CAD build for the part. Positions are in the model's coordinates, mm. Round coordinates to 2 decimals unless told otherwise and drop trailing zeros. Order: outer loops, then holes, each group sorted by start corner. A loop starts at its lowest first (then second) coordinate and runs counter-clockwise, first axis right, second up.
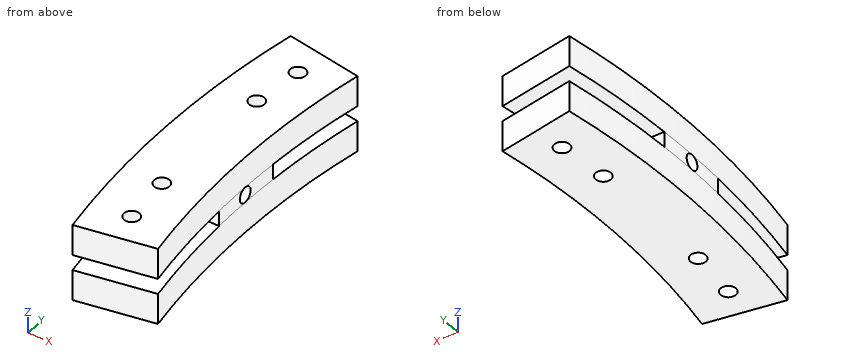
```python
from build123d import *

# Parameters (mm, degrees)
BOSS_EXTRUDE3_DEPTH   = 7.5
CUT_EXTRUDE4_DEPTH    = 1.5
BOSS_EXTRUDE5_DEPTH   = 1.5
SKETCH4_R             = 3
BEARING_HOLE_DEPTH    = 1.25
SHAFT_HOLE_DEPTH      = 33.837885572
SHAFT_HOLE_DEPTH_BACK = 33.837885572
SKETCH7_R             = 1.5
SKETCH3_R             = 1.5
MOUNT_HOLE_DEPTH      = 178.777126728


with BuildPart() as part:
    # Sketch1 → Boss-Extrude3 (new, symmetric)
    with BuildSketch(Plane.XY):
        with BuildLine():
            Line((-157.569240482, 27.783708427), (-172.341356777, 30.388431092))
            ThreePointArc((-172.341356777, 30.388431092), (-175, 0), (-172.341356777, -30.388431092))
            Line((-172.341356777, -30.388431092), (-157.569240482, -27.783708427))
            ThreePointArc((-157.569240482, -27.783708427), (-160, 0), (-157.569240482, 27.783708427))
        make_face()
    extrude(amount=BOSS_EXTRUDE3_DEPTH, both=True)

    # Sketch1_6 → Cut-Extrude4 (cut, symmetric)
    with BuildSketch(Plane.XY):
        with BuildLine():
            Line((-157.569240482, 27.783708427), (-172.341356777, 30.388431092))
            ThreePointArc((-172.341356777, 30.388431092), (-175, 0), (-172.341356777, -30.388431092))
            Line((-172.341356777, -30.388431092), (-157.569240482, -27.783708427))
            ThreePointArc((-157.569240482, -27.783708427), (-160, 0), (-157.569240482, 27.783708427))
        make_face()
    extrude(amount=CUT_EXTRUDE4_DEPTH, both=True, mode=Mode.SUBTRACT)


with BuildPart() as cut_extrude4_piece_1:
    # of the separate pieces the step leaves, piece 1, a body of its own (cut_extrude4_pieces)
    add(part.part.solids().sort_by_distance((-172.341356777, 30.388431092, -1.5))[0])



with BuildPart() as cut_extrude4_piece_2:
    # of the separate pieces the step leaves, piece 2, a body of its own (cut_extrude4_pieces)
    add(part.part.solids().sort_by_distance((-172.341356777, 30.388431092, 7.5))[0])


with BuildPart() as cut_extrude4_piece_1_1:
    add(cut_extrude4_piece_1.part)

    add(cut_extrude4_piece_2.part)  # Boss-Extrude5 merges Cut-Extrude4 piece 2
    # Sketch6 → Boss-Extrude5 (add, symmetric)
    with BuildSketch(Plane.XY):
        with BuildLine():
            Line((-159.824122084, 7.5), (-174.839211849, 7.5))
            ThreePointArc((-174.839211849, 7.5), (-175, 0), (-174.839211849, -7.5))
            Line((-174.839211849, -7.5), (-159.824122084, -7.5))
            ThreePointArc((-159.824122084, -7.5), (-160, 0), (-159.824122084, 7.5))
        make_face()
    extrude(amount=BOSS_EXTRUDE5_DEPTH, both=True)

    # Sketch4 → bearing hole (cut, symmetric)
    with BuildSketch(Plane(origin=(-167.5, 0, 0), x_dir=(0, 0, -1), z_dir=(1, 0, 0))):
        Circle(SKETCH4_R)
    extrude(amount=BEARING_HOLE_DEPTH, both=True, mode=Mode.SUBTRACT)

    # Sketch7 → shaft hole (cut, two sides: drawn at the far end of the back side and taken through both)
    with BuildSketch(Plane(origin=(-167.5, 0, 0), x_dir=(0, 0, -1), z_dir=(1, 0, 0)).offset(-SHAFT_HOLE_DEPTH_BACK)):
        Circle(SKETCH7_R)
    extrude(amount=SHAFT_HOLE_DEPTH + SHAFT_HOLE_DEPTH_BACK, mode=Mode.SUBTRACT)

    # Sketch3 → mount hole (cut, symmetric)
    with BuildSketch(Plane(origin=(0, 0, 0), x_dir=(-1, 0, 0), z_dir=(0, 0, -1))):
        with Locations((165.891323638, 23.158556552)):
            Circle(SKETCH3_R)
        with Locations((166.977667312, 13.217738807)):
            Circle(SKETCH3_R)
    mount_hole = extrude(amount=MOUNT_HOLE_DEPTH, both=True, mode=Mode.SUBTRACT)

    # Mirror1: mount hole across plane
    add(mount_hole.mirror(Plane.ZX), mode=Mode.SUBTRACT)


solid = cut_extrude4_piece_1_1.part
```
1. Pin check, flat tips, straight feed: P1, Ø5, axis at y = 9, z = -5.5, coming from the -X side; P2, Ø4, axis at y = 13.5, z = -3, coming from the -X side; P3, Ø3.5, axis at x = -167, z = 0.5, coming from the +Y side. Stop position of each tip, or through.
2. Cut at D-D, the plane z = 4. Write the cut outline in (x, y), and give its area (3 significant figures).
3. Cut at A-A, the plane y = -9.5. Write the cut outline in (x, z).
4. Drill centre lines: line 1 (Y direction, x = -165.75, z = 3.5); line 2 (Y direction, x = -167, z = 6); line 3 (Z direction, x = -168.25, y = -9). Where is each one in solid material? Low to high.
5. Cut at C-C, the plane y = 9. Write the cut outline in (x, z), and give its area (3 significant figures).
6. Cut at B-B, the plane z = 0. Write the cut outline in (x, y).
Outcome:
1. P1: stops at x = -174.88
1. P2: stops at x = -174.62
1. P3: stops at y = 29.7
2. outline: (-172.34, -30.39) - (-157.57, -27.78) arc R160 cw to (-157.57, 27.78) - (-172.34, 30.39) arc R175 ccw to start; hole circle Ø3 at (-166.98, -13.22); hole circle Ø3 at (-166.98, 13.22); hole circle Ø3 at (-165.89, -23.16); hole circle Ø3 at (-165.89, 23.16)
2. area: 849 mm2
3. outline: (-174.74, -7.5) - (-159.72, -7.5) - (-159.72, -1.5) - (-174.74, -1.5) - close; (-174.74, 1.5) - (-159.72, 1.5) - (-159.72, 7.5) - (-174.74, 7.5) - close
4. line 1: y = -29.23 to -24.65, -21.67 to -14.08, -12.36 to 12.36, 14.08 to 21.67, 24.65 to 29.23
4. line 2: y = -29.45 to -24.17, -22.15 to -14.72, -11.72 to 11.72, 14.72 to 22.15, 24.17 to 29.45
4. line 3: z = -7.5 to -1.5, 1.5 to 7.5
5. outline: (-174.77, -7.5) - (-159.75, -7.5) - (-159.75, -1.5) - (-174.77, -1.5) - close; (-174.77, 1.5) - (-159.75, 1.5) - (-159.75, 7.5) - (-174.77, 7.5) - close
5. area: 180 mm2
6. outline: (-174.99, -1.5) arc R175 ccw to (-174.84, -7.5) - (-159.82, -7.5) arc R160 cw to (-159.99, -1.5) - (-166.25, -1.5) - (-166.25, -3) - (-168.75, -3) - (-168.75, -1.5) - close; (-174.99, 1.5) - (-168.75, 1.5) - (-168.75, 3) - (-166.25, 3) - (-166.25, 1.5) - (-159.99, 1.5) arc R160 cw to (-159.82, 7.5) - (-174.84, 7.5) arc R175 ccw to start
